Part model, mm, in its own coordinate system. A direction names the side the tool comes from. Round coordinates to 2 decimals unless told otherwise and drop trailing zeros. Order: outer loops, then holes, each group sorted by start corner. A loop starts at its lowest first (then second) coordinate and runs counter-clockwise, first axis right, second up. Notation, with made-up numbers: (25.5, -34.5) - (84.5, -34.5) arc R29 ccw to (84.5, -7.5) - close; hole circle Ø10 at (12.5, -15). An arc over 180 degrees is marked (long way). Return JSON: item names as keys, results as strings. Group by question number.
Item 1: Saw through at A-A on z = 4.25. List the corners of the cut face in (x, y), and give its area (3 significant figures).
Item 2: Saw through at B-B on x = -19.5. List the corners of the cut face in (y, z), and give its area (3 significant figures).
Item 3: Saw through at D-D on z = 1.25. List the corners of the cut face in (x, y).
Item 4: Drop flat-ended pins along their axis: pin 1 (9.5 mm diameter, centred on y = 7, z = 8, fed in from +X); pin 2 (2.5 mm diameter, centred on x = -19.5, y = 29, fed in from +Z); pin 3 (1.5 mm diameter, centred on y = 16.5, z = 2, fed in from +X); pin 4 (2.5 mm diameter, centred on x = -6.7, y = 3.96, fed in from +Z). Give the stop position or say it passes through.
Item 5: Two-plate mould, pull along Z, no slides. Class faces 1 (the face through (-12.347, 26, 9)), 2 (the face through (-11.854, 5.613, 7.76)), 3 (the face through (-22, 31, 12.5)): released by +Z, released by -Z, zero draft, split by the parting line, or undercut.
Item 6: Saw through at C-C on y = 5. List the corners of the cut face in (x, z), and give its area (3 significant figures).
Item 7: Probe probe 1 along Y at (x, z) = (-30, 11.5); probe 2 along Y at (x, z) = (-10, 12); probe 3 along X at (y, z) = (6, 9.5). List the from-to ranges inside material, lowest first.
Item 8: Tool access for faces 4 (the face through (-39, 16, 12.5)), 5 (the face through (-26, 0.662, 7)), 6 (the face through (-9.847, 5, 8)), 7 (the face through (-11, 9.162, 8)): list every direction of +Z, -Z, +X, -X, +Y, -Y with a clear straight run to the whole face (end or side of a thin tool).
```python
from build123d import *

# Parameters (mm, degrees)
CROQUIS1_R              = 1.5
SALIENTE_EXTRUIR1_DEPTH = 3
CROQUIS2_W              = 31.2
CROQUIS2_H              = 31.2
CROQUIS2_W_2            = 28.2
CROQUIS2_H_2            = 28.2
SALIENTE_EXTRUIR2_DEPTH = 9.5
CROQUIS4_W              = 28.2
CROQUIS4_H              = 28.2
CROQUIS4_W_2            = 26.2
CROQUIS4_H_2            = 26.2
SALIENTE_EXTRUIR3_DEPTH = 3
CORTAR_EXTRUIR1_REACH   = 69.732
CROQUIS8_W              = 7.2
CROQUIS8_H              = 1
CORTAR_EXTRUIR2_START   = -9.5
CROQUIS9_W              = 5.627722912
CROQUIS9_H              = 14.2
CORTAR_EXTRUIR2_DEPTH   = 9.5
CROQUIS10_W             = 2.5
CROQUIS10_H             = 31.2
SALIENTE_EXTRUIR4_DEPTH = 1
CORTAR_EXTRUIR3_DEPTH   = 3
SALIENTE_EXTRUIR5_START = -2.5
SALIENTE_EXTRUIR5_DEPTH = 2.5


with BuildPart() as part:
    # Croquis1 → Saliente-Extruir1 (new body)
    with BuildSketch(Plane.XY):
        with BuildLine():
            Line((-52.197309417, 4.461883408), (-50.197309417, 4.461883408))
            Line((-50.197309417, 4.461883408), (-44.197309417, 8.461883408))
            Line((-44.197309417, 8.461883408), (-44.197309417, 24.461883408))
            Line((-44.197309417, 24.461883408), (-50.197309417, 28.461883408))
            Line((-50.197309417, 28.461883408), (-52.197309417, 28.461883408))
            ThreePointArc((-52.197309417, 28.461883408), (-56.197309417, 32.461883408), (-52.197309417, 36.461883408))
            Line((-52.197309417, 36.461883408), (-5.197309417, 36.461883408))
            ThreePointArc((-5.197309417, 36.461883408), (-3.075989073, 35.583203752), (-2.197309417, 33.461883408))
            Line((-2.197309417, 33.461883408), (-2.197309417, 26.567434684))
            ThreePointArc((-2.197309417, 26.567434684), (-2.552285621, 25.151860907), (-3.533208828, 24.071283801))
            Line((-3.533208828, 24.071283801), (-7.361410006, 21.519149682))
            ThreePointArc((-7.361410006, 21.519149682), (-8.342333213, 20.438572576), (-8.697309417, 19.022998799))
            Line((-8.697309417, 19.022998799), (-8.697309417, 13.900768017))
            ThreePointArc((-8.697309417, 13.900768017), (-8.342333213, 12.48519424), (-7.361410006, 11.404617134))
            Line((-7.361410006, 11.404617134), (-3.533208828, 8.852483016))
            ThreePointArc((-3.533208828, 8.852483016), (-2.552285621, 7.771905909), (-2.197309417, 6.356332133))
            Line((-2.197309417, 6.356332133), (-2.197309417, -0.538116592))
            ThreePointArc((-2.197309417, -0.538116592), (-3.075989073, -2.659436935), (-5.197309417, -3.538116592))
            Line((-5.197309417, -3.538116592), (-52.197309417, -3.538116592))
            ThreePointArc((-52.197309417, -3.538116592), (-56.197309417, 0.461883408), (-52.197309417, 4.461883408))
        make_face()
        with Locations((-6.697309417, 28.961883408)):
            Circle(CROQUIS1_R, mode=Mode.SUBTRACT)
        with Locations((-52.197309417, 0.461883408)):
            Circle(CROQUIS1_R, mode=Mode.SUBTRACT)
        with Locations((-6.697309417, 3.961883408)):
            Circle(CROQUIS1_R, mode=Mode.SUBTRACT)
        with Locations((-52.197309417, 32.461883408)):
            Circle(CROQUIS1_R, mode=Mode.SUBTRACT)
    extrude(amount=SALIENTE_EXTRUIR1_DEPTH)

    # Croquis2 → Saliente-Extruir2 (add)
    with BuildSketch(Plane.XY.offset(3)):
        with Locations((-25.447309417, 16.261883408)):
            Rectangle(CROQUIS2_W, CROQUIS2_H)
        with Locations((-25.447309417, 16.261883408)):
            Rectangle(CROQUIS2_W_2, CROQUIS2_H_2, mode=Mode.SUBTRACT)
    extrude(amount=SALIENTE_EXTRUIR2_DEPTH)

    # Croquis4 → Saliente-Extruir3 (add)
    with BuildSketch(Plane.XY.offset(7)):
        with Locations((-25.447309417, 16.261883408)):
            Rectangle(CROQUIS4_W, CROQUIS4_H)
        with Locations((-25.447309417, 16.261883408)):
            Rectangle(CROQUIS4_W_2, CROQUIS4_H_2, mode=Mode.SUBTRACT)
    extrude(amount=SALIENTE_EXTRUIR3_DEPTH)

    # Cortar-Barrer1: sweep along a path in Croquis7
    with BuildLine(Plane.XY.offset(10)) as cortar_barrer1_path:
        Line((-39.047309417, 29.861883408), (-11.847309417, 29.861883408))
        Line((-11.847309417, 29.861883408), (-11.847309417, 2.661883408))
        Line((-11.847309417, 2.661883408), (-39.047309417, 2.661883408))
        Line((-39.047309417, 2.661883408), (-39.047309417, 29.861883408))
    # Croquis6 → Cortar-Barrer1 (sweep, cut)
    with BuildSketch(Plane(origin=(0, 3.161883408, 0), x_dir=(-1, 0, 0), z_dir=(0, -1, 0))):
        Polygon((38.547309417, -8.5), (38.547309417, -7), (39.547309417, -7), align=None)
    sweep(path=cortar_barrer1_path.line, transition=Transition.RIGHT, mode=Mode.SUBTRACT)

    # Cortar-Extruir1: up to this plane
    cortar_extruir1_end = Plane(origin=(-39.697309417, 30.361883408, 7), z_dir=(0, -0.8320502943378436, -0.5547001962252293))
    # Croquis8 → Cortar-Extruir1 (cut, up to the surface)
    with BuildSketch(Plane.XY.offset(10), mode=Mode.PRIVATE) as cortar_extruir1_sk1:
        with Locations((-26.947309417, 29.861883408)):
            Rectangle(CROQUIS8_W, CROQUIS8_H)
    cortar_extruir1_tool1 = split(extrude(cortar_extruir1_sk1.sketch, amount=-CORTAR_EXTRUIR1_REACH, mode=Mode.PRIVATE), bisect_by=cortar_extruir1_end, keep=Keep.BOTH, mode=Mode.PRIVATE)
    add(cortar_extruir1_tool1.solids().sort_by_distance((-26.947309, 29.861883, 10))[0], mode=Mode.SUBTRACT)

    # Croquis9 → Cortar-Extruir2 (cut)
    with BuildSketch(Plane.XY.offset(12.5).offset(CORTAR_EXTRUIR2_START)):
        with Locations((-12.661170873, 16.261883408)):
            Rectangle(CROQUIS9_W, CROQUIS9_H)
    extrude(amount=CORTAR_EXTRUIR2_DEPTH, mode=Mode.SUBTRACT)

    # Croquis10 → Saliente-Extruir4 (add)
    with BuildSketch(Plane.XY.offset(12.5)):
        with Locations((-39.797309417, 16.261883408)):
            Rectangle(CROQUIS10_W, CROQUIS10_H)
    extrude(amount=SALIENTE_EXTRUIR4_DEPTH)

    # Croquis12 → Cortar-Extruir3 (cut)
    with BuildSketch(Plane.XY.offset(3)):
        with BuildLine():
            Line((-9.847309417, 31.861883408), (-41.047309417, 31.861883408))
            Line((-41.047309417, 31.861883408), (-41.047309417, 0.661883408))
            Line((-41.047309417, 0.661883408), (-9.847309417, 0.661883408))
            ThreePointArc((-9.847309417, 0.661883408), (-4.614210238, 1.617448149), (-2.197309417, 6.356332133))
            Line((-2.197309417, 6.356332133), (-2.197309417, -17.8731401))
            Line((-2.197309417, -17.8731401), (-65.359464881, -17.8731401))
            Line((-65.359464881, -17.8731401), (-65.359464881, 40.399106007))
            Line((-65.359464881, 40.399106007), (-2.197309417, 40.399106007))
            Line((-2.197309417, 40.399106007), (-2.197309417, 26.567434684))
            ThreePointArc((-2.197309417, 26.567434684), (-4.764439849, 31.03216691), (-9.847309417, 31.861883408))
        make_face()
    extrude(amount=-CORTAR_EXTRUIR3_DEPTH, mode=Mode.SUBTRACT)

    # Croquis13 → Saliente-Extruir5 (add)
    with BuildSketch(Plane.ZY.offset(41.047309417).offset(SALIENTE_EXTRUIR5_START)):
        with BuildLine():
            Line((13.5, 31.861883408), (13.5, 0.661883408))
            ThreePointArc((13.5, 0.661883408), (17.168865325, 16.261883408), (13.5, 31.861883408))
        make_face()
    extrude(amount=SALIENTE_EXTRUIR5_DEPTH)


solid = part.part
```
Filled in:
{
 "1": {"outline": "(-41.05, 0.66) - (-9.85, 0.66) - (-9.85, 9.16) - (-11.35, 9.16) - (-11.35, 2.16) - (-39.55, 2.16) - (-39.55, 30.36) - (-11.35, 30.36) - (-11.35, 23.36) - (-9.85, 23.36) - (-9.85, 31.86) - (-41.05, 31.86) - close", "area": "157 mm^2"},
 "2": {"outline": "(0.66, 0) - (31.86, 0) - (31.86, 12.5) - (30.36, 12.5) - (30.36, 10) - (29.36, 10) - (29.36, 8.5) - (30.36, 7) - (30.36, 3) - (2.16, 3) - (2.16, 7) - (3.16, 8.5) - (3.16, 10) - (2.16, 10) - (2.16, 12.5) - (0.66, 12.5) - close", "area": "127 mm^2"},
 "3": {"outline": "(-41.05, 0.66) - (-9.85, 0.66) arc R6 ccw to (-2.2, 6.36) arc R3 ccw to (-3.53, 8.85) - (-7.36, 11.4) arc R3 cw to (-8.7, 13.9) - (-8.7, 19.02) arc R3 cw to (-7.36, 21.52) - (-3.53, 24.07) arc R3 ccw to (-2.2, 26.57) arc R6 ccw to (-9.85, 31.86) - (-41.05, 31.86) - close; hole circle Ø3 at (-6.7, 3.96); hole circle Ø3 at (-6.7, 28.96)"},
 "4": {"pin 1": "stops at x = -9.85", "pin 2": "stops at z = 10", "pin 3": "stops at x = -8.7", "pin 4": "passes through"},
 "5": {"face 1": "zero draft", "face 2": "undercut", "face 3": "released by +Z"},
 "6": {"outline": "(-41.05, 0) - (-7.78, 0) - (-7.78, 3) - (-9.85, 3) - (-9.85, 12.5) - (-11.35, 12.5) - (-11.35, 10) - (-12.35, 10) - (-12.35, 8.5) - (-11.35, 7) - (-11.35, 3) - (-39.55, 3) - (-39.55, 7) - (-38.55, 8.5) - (-38.55, 10) - (-39.55, 10) - (-39.55, 12.5) - (-38.55, 12.5) - (-38.55, 15.31) - (-41.05, 15.31) - close; (-5.61, 0) - (-2.37, 0) - (-2.37, 3) - (-5.61, 3) - close", "area": "150 mm^2"},
 "7": {"probe 1": "y = 0.66 to 2.16, 30.36 to 31.86", "probe 2": "y = 0.66 to 9.16, 23.36 to 31.86", "probe 3": "x = -41.05 to -38.55, -12.35 to -9.85"},
 "8": {"face 4": "none", "face 5": "+Z, -Z, -X, -Y", "face 6": "+Z, +X, +Y, -Y", "face 7": "+Z, +X"}
}
